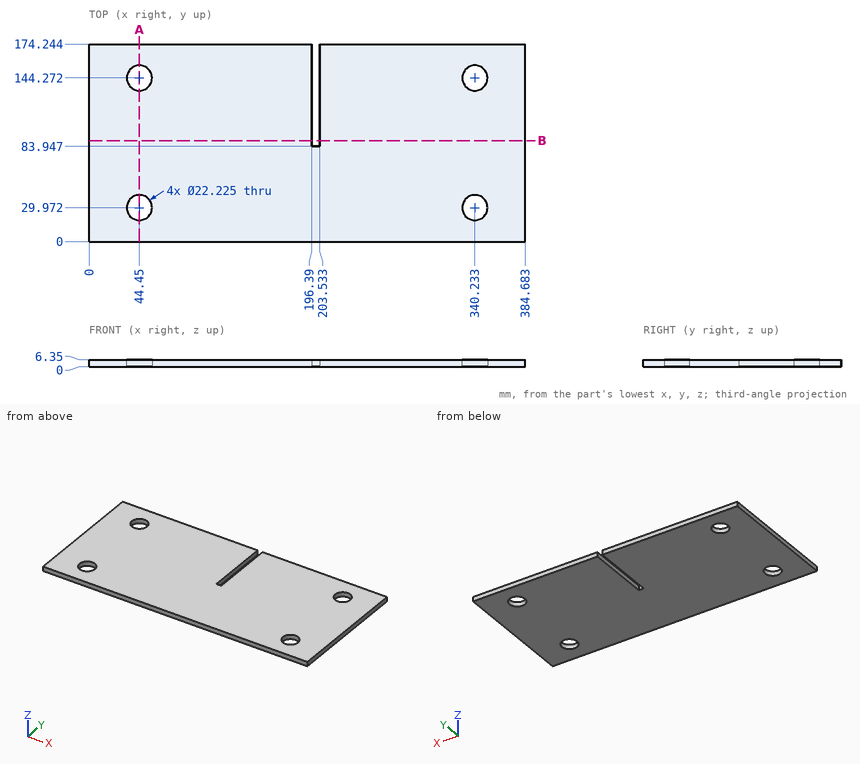
Here's the drawing with two shaded views (mm, measured from the low corner). I have some questions. Coordinates: 2 decimals unless noted, no trailing zeros. Loops run counter-clockwise (first coordinate to the right, second up) from the corner with the lowest first, then second, coordinate; pieces in that order, holes last. Notation, with made-up numbers: (35.5, -22) - (64.5, -22) arc R10 cw to (64.5, -4) - close; hole circle Ø4 at (-3, -1). An arc over 180 degrees is marked (long way). Answer as CSV lines item,"result". Start each with the question number.
1) Suppose I cut it at B-B (y = 89). Please give me the cut outline in (x, z).
2) I need wall thicknesses on line 1 (X direction, y = 30, z = 6.25) (1 decimal); line 2 (Y direction, x = 44.5, z = 3) (1 decimal); line 3 (X direction, y = 148, z = 5.5) (1 decimal). Which ranges of each line are inside material? Lowest first, please. Write a range as from..to.
3) Suppose I cut it at A-A (x = 44.45). Count the separate pieces of the cut face and the enclosed holes in it, plus the area to 3 significant figures.
4) For pin 1 (1.5 mm diameter, centred on x = 297, z = 2.5, fed in from -Y); pin 2 (13.5 mm diameter, centred on x = 44.45, y = 29.972, fed in from +Z), each with a flat end and sliding along its axis, tell me the tip position at first contact or that it passes through.
Check result:
1,outline,"(0, 0) - (196.39, 0) - (196.39, 6.35) - (0, 6.35) - close; (203.53, 0) - (384.68, 0) - (384.68, 6.35) - (203.53, 6.35) - close"
2,line 1,"x = 0..33.3, 55.6..329.1, 351.3..384.7"
2,line 2,"y = 0..18.9, 41.1..133.2, 155.4..174.2"
2,line 3,"x = 0..34, 54.9..196.4, 203.5..329.8, 350.7..384.7"
3,separate pieces,"3"
3,enclosed holes,"0"
3,area,"824 mm²"
4,pin 1,"stops at y = 0"
4,pin 2,"passes through"
